Model file for the job. Use its own axes, mm. Face numbers are marked on the shaded views. Coordinates: 2 decimals unless noted, no trailing zeros. Loops run counter-clockwise (first coordinate to the right, second up) from the corner with the lowest first, then second, coordinate; pieces in that order, holes last.
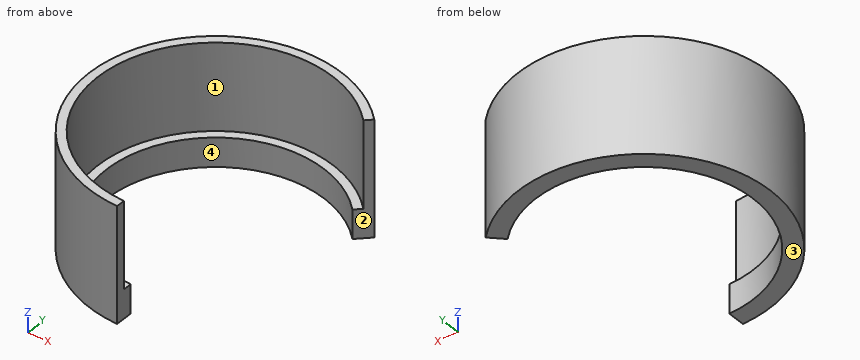
from build123d import *

# Parameters (mm, degrees)
EXTRUDE_1_DEPTH      = 10
EXTRUDE_2_DEPTH      = 30
EXTRUDE_2_DEPTH_BACK = 10


with BuildPart() as part:
    # 草图1 → 凸台-拉伸1 (new body)
    with BuildSketch(Plane.XY):
        with BuildLine():
            Line((0, -40.6), (0, -37.6))
            ThreePointArc((0, -37.6), (-34.737870422, 14.388897057), (26.587214973, 26.587214973))
            Line((26.587214973, 26.587214973), (28.708535316, 28.708535316))
            ThreePointArc((28.708535316, 28.708535316), (-37.50950902, 15.536947354), (0, -40.6))
        make_face()
    extrude(amount=EXTRUDE_1_DEPTH)

    # 草图2 → 凸台-拉伸2 (add, two sides: drawn at the far end of the back side and taken through both)
    with BuildSketch(Plane.XY.offset(10).offset(-EXTRUDE_2_DEPTH_BACK)):
        with BuildLine():
            ThreePointArc((0, -40.6), (-37.50950902, 15.536947354), (28.708535316, 28.708535316))
            Line((28.708535316, 28.708535316), (30.82985566, 30.82985566))
            ThreePointArc((30.82985566, 30.82985566), (-40.281147617, 16.684997651), (0, -43.6))
            Line((0, -43.6), (0, -40.6))
        make_face()
    extrude(amount=EXTRUDE_2_DEPTH + EXTRUDE_2_DEPTH_BACK)


solid = part.part
Q1. Slice it at D-D (x = 21.5). List the corners of the cut face in (y, z).
Answers:
outline: (30.85, 0) - (37.93, 0) - (37.93, 40) - (34.44, 40) - (34.44, 10) - (30.85, 10) - close
Q2. Drill centre lines: line 1 (X direction, y = 0, z = 17.25); line 2 (Y direction, x = -13.5, z = 19.5); line 3 (Z direction, x = -6, y = 38). Where is each one in solid material? Low to high.
Answers:
line 1: x = -43.6 to -40.6
line 2: y = -41.46 to -38.29, 38.29 to 41.46
line 3: z = 0 to 10
Q3. Flat gauge pins, fed straight in: P1, Ø6, axis at y = 25, z = 6, coming from the +X side; P2, Ø12, axis at x = 16, z = 11, coming from the -Y side; P3, Ø21, axis at x = -4.5, y = 19, coming from the +Z side; P4, Ø12, axis at x = 13, z = 10, coming from the -Y side. Where does each tip first touch, or does it go through?
Answers:
P1: stops at x = 28
P2: stops at y = 30.55
P3: passes through
P4: stops at y = 32.45
Q4. Slice it at C-C (z = 7). List the corners of the cut face in (x, y), and give its area (3 significant figures).
Answers:
outline: (0, -43.6) - (0, -37.6) arc R37.6 cw (long way) to (26.59, 26.59) - (30.83, 30.83) arc R43.6 ccw (long way) to start
area: 957 mm2
Q5. Slice it at B-B (y = 0). List the corners of the cut face in (x, z).
Answers:
outline: (-43.6, 0) - (-37.6, 0) - (-37.6, 10) - (-40.6, 10) - (-40.6, 40) - (-43.6, 40) - close
Q6. Slice it at A-A (x = -20). List the corners of the cut face in (y, z).
Answers:
outline: (-38.74, 0) - (-31.84, 0) - (-31.84, 10) - (-35.33, 10) - (-35.33, 40) - (-38.74, 40) - close; (31.84, 0) - (38.74, 0) - (38.74, 40) - (35.33, 40) - (35.33, 10) - (31.84, 10) - close
Q7. Mould opens along Y. For the marked faces 1, 2, 3 and 4 say: +Y half, -Y half, draft (parallel to the pull), parting line (faces both ways), or undercut.
Answers:
face 1: undercut
face 2: -Y half
face 3: draft
face 4: undercut
